Check sheet for the modelled part. Datum: model origin and axes. Units: mm. Face numbers are marked on the shaded views. A direction names the side the tool comes from. Round coordinates to 2 decimals unless told otherwise and drop trailing zeros. Write each loop counter-clockwise with the first axis right and the second up, starting at its lowest first coordinate (ties: lowest second). Pieces come first, ordered by that corner, then holes. Notation, with made-up numbers: (55, 57) -> (104, 57) arc R27 ccw to (104, 90) -> close; hole circle Ø11 at (51.25, -0.75). An arc over 180 degrees is marked (long way). One line per item, written item: value.
Autodesk Inventor part; units mm, degrees
ref_plane "YZ Plane" through (0, 0, 0) normal (1, 0, 0) x (0, 1, 0)
ref_plane "XZ Plane" through (0, 0, 0) normal (0, 1, 0) x (-1, 0, 0)
ref_plane "XY Plane" through (0, 0, 0) normal (0, 0, 1) x (1, 0, 0)
sketch "Sketch1" plane through (0, 0, 0) normal (0, 0, 1) x (1, 0, 0)
  line L0 (-37, -30) -> (-37, 0)
  line L1 (-37, 0) -> (37, 0)
  line L2 (37, 0) -> (37, -30)
  point P0 (0, 0)
  point P1 (0, 0)
  dimension "d0" = 30
  dimension "d1" = 74
contour flange "Contour Flange1" sketch "Sketch1" thickness 3 bend radius 3 width 30 along (0, 0, 1) mid plane no both sides no wall seen from (-37, -15, 0) lies toward (1, 0, 0) curves L0 L1 L2
bend "Bend1"
corner "Corner1"
equation "\"d4\" = Thickness"
equation "\"d5\" = BendReliefWidth"
equation "\"d6\" = BendReliefDepth"
equation "\"d7\" = MinimumRemnant"
equation "\"d8\" = TransitionRadius"
equation "\"d10\" = BendRadius"
equation "\"d12\" = CornerReliefSize"
equation "\"d13\" = GapSize"
equation "\"d14\" = JacobiRadiusSize"
equation "\"BendRadius\" = Thickness"
equation "\"BendReliefWidth\" = Thickness"
equation "\"BendReliefDepth\" = 0.5 * Thickness"
equation "\"CornerReliefSize\" = 4 * Thickness"
equation "\"MinimumRemnant\" = 2 * Thickness"
equation "\"TransitionRadius\" = BendRadius"
equation "\"JacobiRadiusSize\" = BendRadius"
equation "\"GapSize\" = Thickness"
properties part number "ДМФ 01 55 Усилитель кассеты"
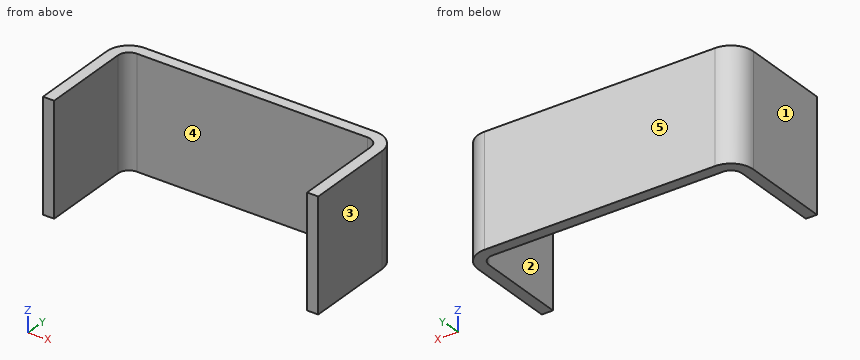
Item 1: Sectioned sample at A-A (y = -17). Enter the section's corners in (x, z).
Result set:
outline: (-37, 0) -> (-34, 0) -> (-34, 30) -> (-37, 30) -> close; (34, 0) -> (37, 0) -> (37, 30) -> (34, 30) -> close
Item 2: Tool access check on the marked faces 1 and 2. Record the directions out of +Z, -Z, +X, -X, +Y, -Y that give a thin tool (end or side, any length) a straight path to the whole face; none if there is none.
Result set:
face 1: +Z, -Z, -X, +Y, -Y
face 2: +Z, -Z, -Y
Item 3: Sectioned sample at B-B (z = 10.75). Enter the section's corners in (x, y), then the cut area to 3 significant figures.
Result set:
outline: (-37, -30) -> (-34, -30) -> (-34, -6) arc R3 cw to (-31, -3) -> (31, -3) arc R3 cw to (34, -6) -> (34, -30) -> (37, -30) -> (37, -6) arc R6 ccw to (31, 0) -> (-31, 0) arc R6 ccw to (-37, -6) -> close
area: 372 mm^2
Item 4: Release check for a two-part mould opening along X. For the marked faces 3, 4 and 5 record: pulls with the +X half, pulls with the -X half, needs draft (parallel to the pull), parting line crosses it, or undercut.
Result set:
face 3: pulls with the +X half
face 4: undercut
face 5: needs draft
Item 5: Depth check by flat-ended pin: pin 1 (9 mm diameter, centred on x = -11, z = 11.5, fed in from -Y). Enter the tip coordinate at first touch or a pass-through.
Result set:
pin 1: y = -3
Item 6: Material ranges on line 1 along X through (y, z) = (-13.25, 12.75); line 2 along Y through (x, z) = (13.5, 13.5); line 3 along X through (y, z) = (-4, 2.25), recorded low to high.
Result set:
line 1: -37 to -34, 34 to 37
line 2: -3 to 0
line 3: -36.66 to -33.24, 33.24 to 36.66
Item 7: Sectioned sample at C-C (x = 25.5). Enter the section's corners in (y, z), then the cut area to 3 significant figures.
Result set:
outline: (-3, 0) -> (0, 0) -> (0, 30) -> (-3, 30) -> close
area: 90.0 mm^2
